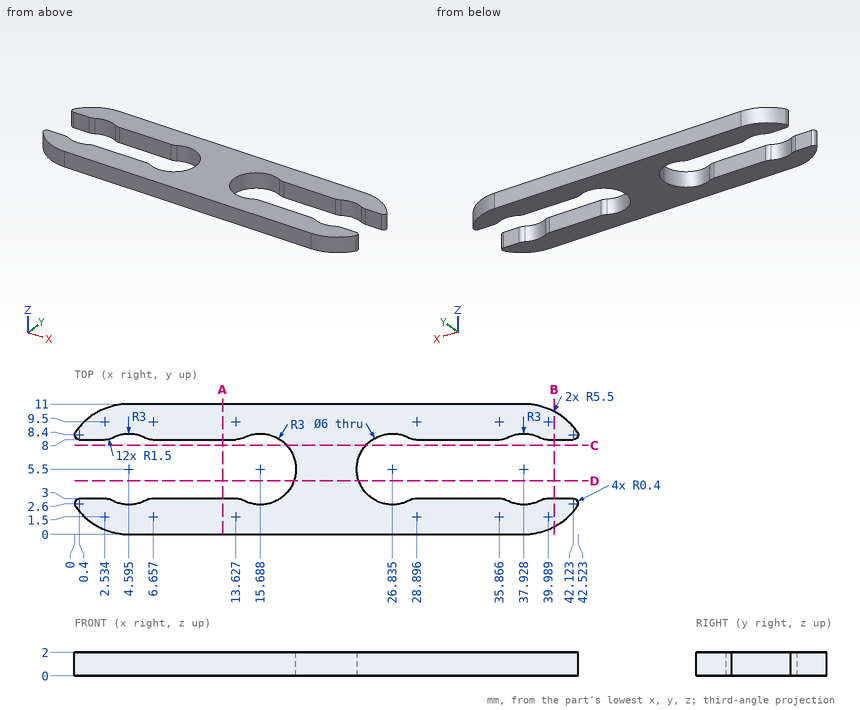
For this review, use the dimensioned drawing (mm, ordinates from the lowest corner) and the shaded views. Round coordinates to 2 decimals unless told otherwise and drop trailing zeros. Write each loop counter-clockwise with the first axis right and the second up, starting at its lowest first coordinate (ties: lowest second). Pieces come first, ordered by that corner, then holes. Notation, with made-up numbers: (11.5, 39.25) -> (48.5, 39.25) arc R13 ccw to (48.5, 51.25) -> close; hole circle Ø3 at (52.5, -24). An arc over 180 degrees is marked (long way). Use CSV: the item, a comma, the result in double quotes.
(1) Consider section B-B, the plane x = 40.5. Give the boundary of the cut face in (y, z).
Computed values:
outline,"(0.64, 0) -> (3, 0) -> (3, 2) -> (0.64, 2) -> close; (8, 0) -> (10.36, 0) -> (10.36, 2) -> (8, 2) -> close"
(2) Consider section C-C, the plane y = 7.5. Give the boundary of the cut face in (x, z) (1 decimal).
Computed values:
outline,"(17.9, 0) -> (24.6, 0) -> (24.6, 2) -> (17.9, 2) -> close"
(3) To check wall thickness, follow L1, parallel to Y at x = 11.5, z = 0.35; L2, parallel to X at y = 8.25, z = 1.2 (1 decimal); L3, parallel to Y at x = 16.5, z = 1.35. State the ranges of each line that lie inside material, in increasing order. Write a range as [from, to].
Computed values:
L1,"[0, 3], [8, 11]"
L2,"[0, 3.4], [5.8, 14.5], [16.9, 25.6], [28, 36.7], [39.1, 42.5]"
L3,"[0, 2.61], [8.39, 11]"
(4) Clearance check with flat-ended pins moving along their axes: P1, Ø0.6, axis at x = 1.5, z = 1.5, coming from the -Y side; P2, Ø1, axis at x = 1, z = 1, coming from the +Y side. State where each tip first meets the part, or that it passes through.
Computed values:
P1,"y = 0.76"
P2,"y = 10.05"
(5) Consider section D-D, the plane y = 4.5. Give the boundary of the cut face in (x, z).
Computed values:
outline,"(18.52, 0) -> (24.01, 0) -> (24.01, 2) -> (18.52, 2) -> close"
(6) Consider section A-A, the plane x = 12.5. Give the boundary of the cut face in (y, z), plus the area to 3 significant figures.
Computed values:
outline,"(0, 0) -> (3, 0) -> (3, 2) -> (0, 2) -> close; (8, 0) -> (11, 0) -> (11, 2) -> (8, 2) -> close"
area,"12.0 mm²"
